Print and shaded views of the part. All mm, measured from the part's lowest x, y and z. Round coordinates to 2 decimals unless told otherwise and drop trailing zeros. Write each loop counter-clockwise with the first axis right and the second up, starting at its lowest first coordinate (ties: lowest second). Pieces come first, ordered by that corner, then holes. Notation, with made-up numbers: (-1, -2) - (5, -2) arc R18 cw to (5, 28) - close; hole circle Ø9 at (-32.5, 74). An arc over 180 degrees is marked (long way). One line per item, written item: value.
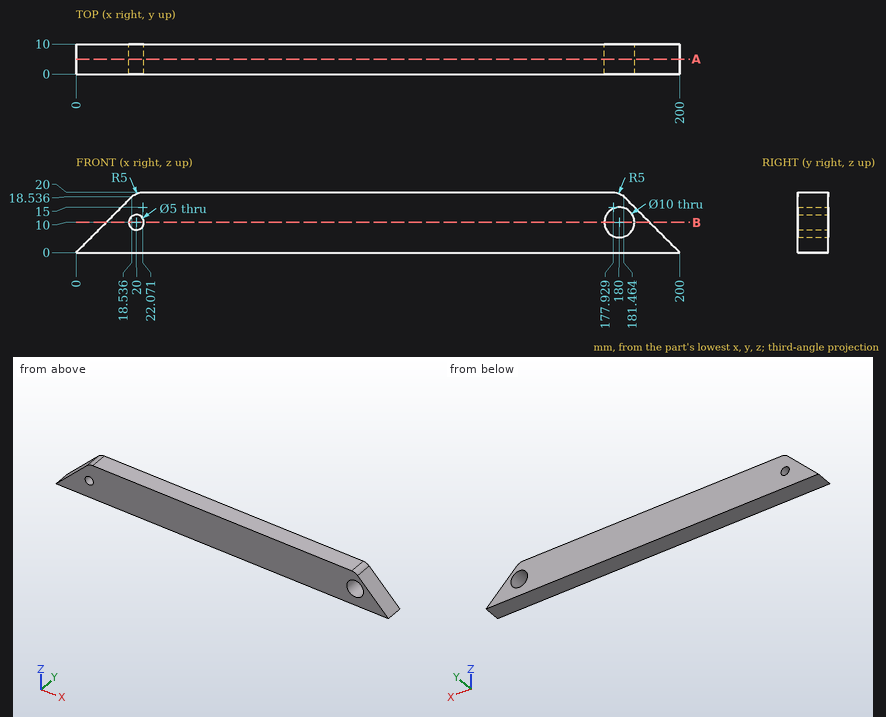
1. Wall check: probe 1 along X at (y, z) = (6, 9); probe 2 along Z at (x, y) = (180, 7); probe 3 along X at (y, z) = (1.25, 6). Give the ranges that are in metal, low to high. Write a range as [from, to].
Report:
probe 1: [9, 17.71], [22.29, 175.1], [184.9, 191]
probe 2: [0, 5], [15, 19.55]
probe 3: [6, 177], [183, 194]
2. Band-saw the part on A-A on y = 5. State how many separate pieces and enclosed holes the cut face has, plus the area to 3 significant figures.
Report:
separate pieces: 1
enclosed holes: 2
area: 3,500 mm²
3. Drop flat-ended pins along their axis: pin 1 (4 mm diameter, centred on y = 4, z = 9.5, fed in from +X); pin 2 (2 mm diameter, centred on y = 6.5, z = 13.5, fed in from -X); pin 3 (6 mm diameter, centred on y = 4.5, z = 6, fed in from +X). Give the stop position or say it passes through.
Report:
pin 1: x = 192.5
pin 2: x = 12.5
pin 3: x = 197
4. Band-saw the part on B-B on z = 10. Write the cut outline in (x, y).
Report:
outline: (10, 0) - (17.5, 0) - (17.5, 10) - (10, 10) - close; (22.5, 0) - (175, 0) - (175, 10) - (22.5, 10) - close; (185, 0) - (190, 0) - (190, 10) - (185, 10) - close
